For this review, take the finished solid that the model builds, in its own axes (mm). Face numbers are marked on the shaded views. A direction names the side the tool comes from. Give positions to 0.01 mm unless a question says otherwise; leave off trailing zeros. Order: outer loops, then holes, each group sorted by start corner. A loop starts at its lowest first (then second) coordinate and runs counter-clockwise, first axis right, second up. Notation, with made-up numbers: (89.5, 86) - (143.5, 86) arc R19 ccw to (143.5, 98) - close; hole circle Ø4 at (34.5, 82). An arc over 180 degrees is marked (long way). One line per item, written item: value.
Autodesk Inventor part; units mm, degrees
ref_plane "YZ Plane" through (0, 0, 0) normal (1, 0, 0) x (0, 1, 0)
ref_plane "XZ Plane" through (0, 0, 0) normal (0, 1, 0) x (-1, 0, 0)
ref_plane "XY Plane" through (0, 0, 0) normal (0, 0, 1) x (1, 0, 0)
sketch "Sketch1" plane through (0, 0, 0) normal (0, 0, 1) x (1, 0, 0)
  arc A0 (-4.8, 0.55) -> (-5.6, -0.25) centre (-4.8, -0.25) ccw
  line L0 (-5.6, -2.6349) -> (-5.6, -0.25)
  arc A1 (-5.6, -2.6349) -> (-5.3449, -3.2206) centre (-4.8, -2.6349) ccw
  arc A2 (-5.1931, -3.4997) -> (-5.3449, -3.2206) centre (-5.6855, -3.5867) ccw
  line L1 (-5.1931, -3.4997) -> (-4.6759, -3.7348)
  line L2 (-4.5, -7.45) -> (-4.5, -4.0079)
  line L3 (4.5, -7.45) -> (-4.5, -7.45)
  line L4 (4.5, -3.9927) -> (4.5, -7.45)
  line L5 (4.7986, -3.679) -> (5.1931, -3.4997)
  arc A3 (5.3449, -3.2206) -> (5.1931, -3.4997) centre (5.6855, -3.5867) ccw
  arc A4 (5.3449, -3.2206) -> (5.6, -2.6349) centre (4.8, -2.6349) ccw
  line L6 (5.6, -2.6349) -> (5.6, -0.25)
  arc A5 (5.6, -0.25) -> (4.8, 0.55) centre (4.8, -0.25) ccw
  line L7 (-4.8, 0.55) -> (4.8, 0.55)
  line L8 (-4.1, -3.65) -> (-4.731, -3.3632)
  arc A6 (-5.2, -2.6349) -> (-4.731, -3.3632) centre (-4.4, -2.6349) ccw
  line L9 (-5.2, -2.6349) -> (-5.2, -0.65)
  arc A7 (-4.4, 0.15) -> (-5.2, -0.65) centre (-4.4, -0.65) ccw
  line L10 (-4.4, 0.15) -> (4.4, 0.15)
  arc A8 (5.2, -0.65) -> (4.4, 0.15) centre (4.4, -0.65) ccw
  line L11 (5.2, -2.6349) -> (5.2, -0.65)
  arc A9 (4.731, -3.3632) -> (5.2, -2.6349) centre (4.4, -2.6349) ccw
  line L12 (4.731, -3.3632) -> (4.1, -3.65)
  line L13 (4.1, -7.05) -> (4.1, -3.65)
  line L14 (-4.1, -7.05) -> (4.1, -7.05)
  line L15 (-4.1, -3.65) -> (-4.1, -7.05)
  line L16 (-4, -6.95) -> (4, -6.95)
  line L17 (4, -6.95) -> (4, -3.5856)
  arc A10 (5.1, -0.65) -> (4.4, 0.05) centre (4.4, -0.65) ccw
  line L18 (5.1, -2.6349) -> (5.1, -0.65)
  line L19 (4.4, 0.05) -> (-4.4, 0.05)
  line L20 (4, -3.5856) -> (4.6897, -3.2721)
  arc A11 (4.6897, -3.2721) -> (5.1, -2.6349) centre (4.4, -2.6349) ccw
  line L21 (-4, -6.95) -> (-4, -3.5856)
  line L22 (-4, -3.5856) -> (-4.6897, -3.2721)
  line L23 (-5.1, -2.6349) -> (-5.1, -0.65)
  arc A12 (-5.1, -2.6349) -> (-4.6897, -3.2721) centre (-4.4, -2.6349) ccw
  arc A13 (-4.4, 0.05) -> (-5.1, -0.65) centre (-4.4, -0.65) ccw
  arc A14 (4.7372, -3.6993) -> (4.7986, -3.679) centre (4.6744, -3.4059) ccw
  arc A15 (4.7372, -3.6993) -> (4.5, -3.9927) centre (4.8, -3.9927) ccw
  arc A16 (-4.5, -4.0079) -> (-4.6759, -3.7348) centre (-4.8, -4.0079) ccw
  point P0 (0, 0)
  dimension "d1" = 0.1
  dimension "d2" = 0.1
  dimension "d3" = 0.1
  dimension "d4" = 0.1
  dimension "d5" = 0.1
  dimension "d7" = 0.1
  dimension "d8" = 0.1
  dimension "d9" = 0.1
  dimension "d10" = 0.1
  dimension "d11" = 0.1
  dimension "d13" = 0.1
  dimension "d15" = 0.1
extrude "Extrusion1" add sketch "Sketch1" along normal blind 0.4 contours L21 L22 A12 L23 A13 L19 A10 L18 A11 L20 L17 L16
sketch "Sketch2" plane through (0, 0, 0.4) normal (0, 0, 1) x (1, 0, 0)
  line L0 (0.15, -3.5039) -> (-2.35, -3.5039)
  line L1 (-2.35, -3.5039) -> (-2.35, -1.0039)
  line L2 (-2.35, -1.0039) -> (0.15, -1.0039)
  line L3 (0.15, -1.0039) -> (0.15, -3.5039)
  line L4 (4.4, 0.05) -> (-4.4, 0.05)
  line L5 (-5.1, -0.65) -> (-5.1, -2.6349)
  line L6 (5.1, -2.6349) -> (5.1, -0.65)
  point P0 (0, 0)
  dimension "d18" = 1.0539
  dimension "d19" = 2.75
  dimension "d21" = 2.5
  dimension "d22" = 4.95
  dimension "d23" = 2.5
extrude "Extrusion2" cut sketch "Sketch2" against normal up to surface (0.4 mm away)
sketch "Sketch3" plane through (0, 0, 0) normal (0, 0, -1) x (-1, 0, 0)
  line L0 (-1.0895, -3.95) -> (2.3023, -3.95)
  line L1 (2.3023, -3.95) -> (2.3023, -4.35)
  line L2 (2.3023, -4.35) -> (-1.0895, -4.35)
  line L3 (-1.0895, -4.35) -> (-1.0895, -3.95)
  line L4 (-4.4, 0.05) -> (4.4, 0.05)
  point P0 (0, 0)
  dimension "d28" = 4
  dimension "d29" = 0.4
extrude "Extrusion3" add sketch "Sketch3" along normal blind 3
equation "\"d2\" = d1"
equation "\"d3\" = d1"
equation "\"d4\" = d2"
equation "\"d5\" = d1"
equation "\"d7\" = d4"
equation "\"d8\" = d2"
equation "\"d9\" = d1"
equation "\"d10\" = d9"
equation "\"d11\" = d10"
properties part number "top_closure"
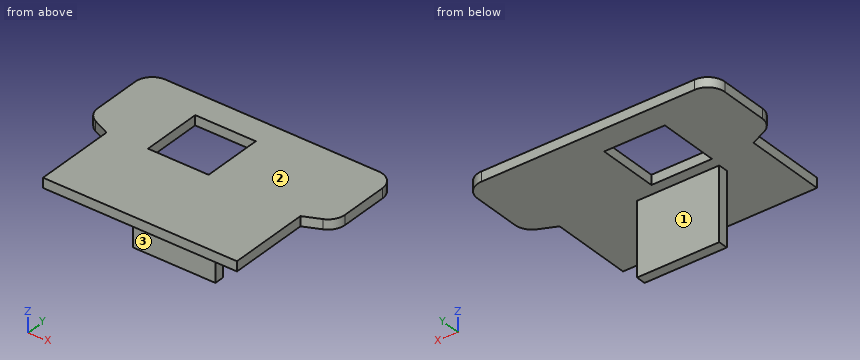
(1) Take a section at D-D (z = -0.3). Write out the cut boundary in (x, y), then the cut area to 3 significant figures.
Answers below:
outline: (-2.3, -4.35) - (1.09, -4.35) - (1.09, -3.95) - (-2.3, -3.95) - close
area: 1.36 mm^2
(2) Take a section at C-C (y = -4.5). Write out the cut boundary in (x, z).
Answers below:
outline: (-4, 0) - (4, 0) - (4, 0.4) - (-4, 0.4) - close
(3) For P1, Ø1.5, axis at x = -1.5, z = -1.5, coming from the -Y side; P2, Ø2, axis at x = 3, y = -4, coming from the -Z side, all flat-tipped, find the tip position at first contact; note any pin that passes through.
Answers below:
P1: stops at y = -4.35
P2: stops at z = 0
(4) Machinability: for the marked faces 1, 2 and 3, which of the approach directions +Z, -Z, +X, -X, +Y, -Y give a long, thin tool a straight path to every point of the face, cutting with its end or side? Answer none if there is none.
Answers below:
face 1: -Z, +X, -X, +Y
face 2: +Z, +X, -X, +Y, -Y
face 3: -Z, +X, -X, -Y
(5) Take a section at A-A (y = -1.25). Write out the cut boundary in (x, z).
Answers below:
outline: (-5.1, 0) - (-2.35, 0) - (-2.35, 0.4) - (-5.1, 0.4) - close; (0.15, 0) - (5.1, 0) - (5.1, 0.4) - (0.15, 0.4) - close
(6) Wall thickness on line 1 (Y direction, x = 0.75, z = -2.55); line 2 (Z direction, x = -3.25, y = -1.5); line 3 (X direction, y = -4, z = -1.1): over which ranges is each line inside the solid? List them lowest first. Write a range as from..to.
Answers below:
line 1: y = -4.35..-3.95
line 2: z = 0..0.4
line 3: x = -2.3..1.09
(7) Take a section at B-B (x = -1.5). Write out the cut boundary in (y, z), then the cut area to 3 significant figures.
Answers below:
outline: (-6.95, 0) - (-4.35, 0) - (-4.35, -3) - (-3.95, -3) - (-3.95, 0) - (-3.5, 0) - (-3.5, 0.4) - (-6.95, 0.4) - close; (-1, 0) - (0.05, 0) - (0.05, 0.4) - (-1, 0.4) - close
area: 3.00 mm^2
